Input: part model. Units: mm. Frame: model coordinates. A direction names the side the tool comes from. Coordinates: 2 decimals unless noted, no trailing zeros. Write each loop counter-clockwise with the first axis right and the second up, starting at its lowest first coordinate (ties: lowest second). Pieces come first, ordered by that corner, then holes. Notation, with made-up numbers: (40, 37.25) - (79, 37.25) arc R34 cw to (79, 76.25) - close; hole circle Ø11 at (44, -33). An arc over 180 degrees is marked (long way). One line per question, with ' | ' between items. Start each with the question number.
1) Reachability of faces 5 (the cylindrical face through (-1.55, 95.59, 14.84)), 6 (the cylindrical face through (13.836, 0.764, 7.924)) from +Z, -Z, +X, -X, +Y, -Y: full face, straight path, thin tool, end or side. Return the list, or none.
2) Section query A-A on y = 32.5. Return loops of the section in (x, z), and give its area (3 significant figures).
3) First-contact query: P1, Ø5, axis at y = 21.5, z = -6.5, coming from the -X side; P2, Ø2, axis at y = 54.5, z = 5, coming from the -X side; P3, Ø2, axis at x = -6, z = 3.5, coming from the +Y side. Flat tips, straight axial feed; report the tip coordinate or a pass-through.
4) Line query: line 1 (X direction, y = 49, z = 0); line 2 (Z direction, x = 3, y = 36.5); line 3 (Z direction, x = 14, y = 41). Output: solid intervals per line, ascending.
5) Draft query along Z for faces 1 (the cylindrical face through (-0.06, 0.76, -15.94)), 2 (the cylindrical face through (9.351, 49.811, 16.372)), 3 (the flat face through (-15.5, 98.425, -2.6)), 4 (the flat face through (0, 12.7, 0)). Return one class per face: released by +Z, released by -Z, zero draft, split by the parting line, or undercut.
```python
from build123d import *

# Parameters (mm, degrees)
BOSS_EXTRUDE1_DEPTH      = 98.425
SKETCH3_R                = 15.478125
CUT_EXTRUDE1_DEPTH       = 85.725
FILLET1_R                = 1.27
FILLET2_R                = 2.54
FILLET3_R                = 2.54
BOSS_EXTRUDE3_DEPTH      = 0.79375
BOSS_EXTRUDE3_DEPTH_BACK = 3.175
SKETCH7_R                = 1.5875
CUT_EXTRUDE2_START       = -0.635
SKETCH8_R                = 1.5875
CUT_EXTRUDE2_DEPTH       = 0.635
FILLET4_R                = 1.524
FILLET5_R                = 0.254


with BuildPart() as part:
    # Sketch2 → Boss-Extrude1 (new body)
    with BuildSketch(Plane(origin=(0, 0, 0), x_dir=(1, 0, 0), z_dir=(0, 1, 0))):
        Polygon((9.562214756, -16.704101823), (19.247283904, -0.070930017), (9.685069148, 16.633171806), (-9.562214756, 16.704101823), (-19.247283904, 0.070930017), (-9.685069148, -16.633171806), align=None)
    extrude(amount=BOSS_EXTRUDE1_DEPTH)

    # Sketch3 → Cut-Extrude1 (cut)
    with BuildSketch(Plane(origin=(0, 98.425, 0), x_dir=(1, 0, 0), z_dir=(0, 1, 0))):
        with Locations(Location((0, 0, 0), (0, 0, 270))):
            Circle(SKETCH3_R)
    extrude(amount=-CUT_EXTRUDE1_DEPTH, mode=Mode.SUBTRACT)

    # Fillet1
    fillet1_edges = [part.edges().sort_by_distance(p)[0] for p in [
        (0, 12.7, -15.478125),
    ]]
    fillet(fillet1_edges, radius=FILLET1_R)

    # Fillet2
    fillet2_edges = [part.edges().sort_by_distance(p)[0] for p in [
        (-14.466176526, 0, 8.281120895),
        (-14.40474933, 0, -8.38751592),
        (0.061427196, 0, -16.668636815),
        (14.466176526, 0, -8.281120895),
        (14.40474933, 0, 8.38751592),
        (-0.061427196, 0, 16.668636815),
    ]]
    fillet(fillet2_edges, radius=FILLET2_R)

    # Fillet3
    # the kernel refuses this fillet: 2.54 mm, written as the material it takes off along each edge
    with BuildSketch(Plane(origin=(-16.314364452, 2.54, -0.060121633), x_dir=(-0.8678621088062781, 0, 0.49680515305129436), z_dir=(0, -1, 0))) as fillet3_piece_1_section:
        Polygon((0, 0), (FILLET3_R, 0), (FILLET3_R, FILLET3_R * 0.57735026919), (FILLET3_R * 0.5, FILLET3_R * 0.866025403784), align=None)
    fillet3_piece_1 = extrude(amount=FILLET3_R, mode=Mode.PRIVATE)
    fillet3_piece_1 = fillet3_piece_1 - Plane(origin=(-16.314364452, 2.54, -0.060121633), x_dir=(0.9999932097338184, 0, 0.003685171129701924), z_dir=(0, -1, 0)) * Sphere(FILLET3_R, mode=Mode.PRIVATE)
    add(fillet3_piece_1, mode=Mode.SUBTRACT)
    with BuildSketch(Plane(origin=(-8.105115364, 2.54, -14.158714879), x_dir=(0.003685171129702339, 0, -0.9999932097338186), z_dir=(0, -1, 0))) as fillet3_piece_2_section:
        Polygon((0, 0), (FILLET3_R, 0), (FILLET3_R, -FILLET3_R * 0.57735026919), (FILLET3_R * 0.5, -FILLET3_R * 0.866025403784), align=None)
    fillet3_piece_2 = extrude(amount=FILLET3_R, mode=Mode.PRIVATE)
    fillet3_piece_2 = fillet3_piece_2 - Plane(origin=(-8.105115364, 2.54, -14.158714879), x_dir=(0.49680515305129425, 0, 0.867862108806278), z_dir=(0, -1, 0)) * Sphere(FILLET3_R, mode=Mode.PRIVATE)
    add(fillet3_piece_2, mode=Mode.SUBTRACT)
    with BuildSketch(Plane(origin=(-8.209249088, 2.54, 14.098593245), x_dir=(-0.003685171129702708, 0, 0.9999932097338186), z_dir=(0, -1, 0))) as fillet3_piece_3_section:
        Polygon((0, 0), (FILLET3_R, 0), (FILLET3_R, FILLET3_R * 0.57735026919), (FILLET3_R * 0.5, FILLET3_R * 0.866025403784), align=None)
    fillet3_piece_3 = extrude(amount=FILLET3_R, mode=Mode.PRIVATE)
    fillet3_piece_3 = fillet3_piece_3 - Plane(origin=(-8.209249088, 2.54, 14.098593245), x_dir=(0.5031880566825245, 0, -0.8641769376765759), z_dir=(0, -1, 0)) * Sphere(FILLET3_R, mode=Mode.PRIVATE)
    add(fillet3_piece_3, mode=Mode.SUBTRACT)
    with BuildSketch(Plane(origin=(8.209249088, 2.54, -14.098593245), x_dir=(0.8678621088062781, 0, -0.49680515305129436), z_dir=(0, -1, 0))) as fillet3_piece_4_section:
        Polygon((0, 0), (FILLET3_R, 0), (FILLET3_R, -FILLET3_R * 0.57735026919), (FILLET3_R * 0.5, -FILLET3_R * 0.866025403784), align=None)
    fillet3_piece_4 = extrude(amount=FILLET3_R, mode=Mode.PRIVATE)
    fillet3_piece_4 = fillet3_piece_4 - Plane(origin=(8.209249088, 2.54, -14.098593245), x_dir=(-0.5031880566825243, 0, 0.8641769376765759), z_dir=(0, -1, 0)) * Sphere(FILLET3_R, mode=Mode.PRIVATE)
    add(fillet3_piece_4, mode=Mode.SUBTRACT)
    with BuildSketch(Plane(origin=(8.105115364, 2.54, 14.158714879), x_dir=(0.8641769376765761, 0, 0.5031880566825242), z_dir=(0, -1, 0))) as fillet3_piece_5_section:
        Polygon((0, 0), (FILLET3_R, 0), (FILLET3_R, FILLET3_R * 0.57735026919), (FILLET3_R * 0.5, FILLET3_R * 0.866025403784), align=None)
    fillet3_piece_5 = extrude(amount=FILLET3_R, mode=Mode.PRIVATE)
    fillet3_piece_5 = fillet3_piece_5 - Plane(origin=(8.105115364, 2.54, 14.158714879), x_dir=(-0.4968051530512941, 0, -0.8678621088062782), z_dir=(0, -1, 0)) * Sphere(FILLET3_R, mode=Mode.PRIVATE)
    add(fillet3_piece_5, mode=Mode.SUBTRACT)
    with BuildSketch(Plane(origin=(16.314364452, 2.54, 0.060121633), x_dir=(0.8641769376765761, 0, 0.5031880566825242), z_dir=(0, -1, 0))) as fillet3_piece_6_section:
        Polygon((0, 0), (FILLET3_R, 0), (FILLET3_R, -FILLET3_R * 0.57735026919), (FILLET3_R * 0.5, -FILLET3_R * 0.866025403784), align=None)
    fillet3_piece_6 = extrude(amount=FILLET3_R, mode=Mode.PRIVATE)
    fillet3_piece_6 = fillet3_piece_6 - Plane(origin=(16.314364452, 2.54, 0.060121633), x_dir=(-0.9999932097338184, 0, -0.003685171129701988), z_dir=(0, -1, 0)) * Sphere(FILLET3_R, mode=Mode.PRIVATE)
    add(fillet3_piece_6, mode=Mode.SUBTRACT)
    with BuildSketch(Plane(origin=(-9.685069148, 2.54, 16.633171806), x_dir=(0.9999932097338186, 0, 0.0036851711297037465), z_dir=(0, 1, 0)), Plane(origin=(-19.247283904, 2.54, -0.070930017), x_dir=(0.49680515305129397, 0, 0.8678621088062782), z_dir=(0, 1, 0)), Plane(origin=(9.562214756, 2.54, 16.704101823), x_dir=(0.5031880566825245, 0, -0.8641769376765758), z_dir=(0, 1, 0))) as fillet3_piece_7:
        with BuildLine():
            CenterArc((FILLET3_R * 0.57735026919, FILLET3_R), FILLET3_R, 210, 60)
            Line((-FILLET3_R * 0.288675134595, FILLET3_R * 0.5), (0, 0))
            Line((0, 0), (FILLET3_R * 0.57735026919, 0))
        make_face()
    extrude(amount=99.551174209, mode=Mode.SUBTRACT)
    with BuildSketch(Plane(origin=(-9.562214756, 2.54, -16.704101823), x_dir=(0.9999932097338186, 0, 0.003685171129701324), z_dir=(0, 1, 0)), Plane(origin=(9.685069148, 2.54, -16.633171806), x_dir=(0.4968051530512946, 0, 0.8678621088062779), z_dir=(0, 1, 0)), Plane(origin=(19.247283904, 2.54, 0.070930017), x_dir=(-0.503188056682524, 0, 0.8641769376765761), z_dir=(0, 1, 0))) as fillet3_piece_8:
        with BuildLine():
            CenterArc((FILLET3_R * 0.57735026919, -FILLET3_R), FILLET3_R, 90, 60)
            Line((-FILLET3_R * 0.288675134595, -FILLET3_R * 0.5), (0, 0))
            Line((0, 0), (FILLET3_R * 0.57735026919, 0))
        make_face()
    extrude(amount=99.551174209, mode=Mode.SUBTRACT)

    # Sketch7 → Boss-Extrude3 (add, two sides: drawn at the far end of the back side and taken through both)
    with BuildSketch(Plane.XY.offset(15.478125).offset(-BOSS_EXTRUDE3_DEPTH_BACK)):
        with Locations(Location((0, 95.25, 0), (0, 0, 270))):
            Circle(SKETCH7_R)
    extrude(amount=BOSS_EXTRUDE3_DEPTH + BOSS_EXTRUDE3_DEPTH_BACK)

    # Sketch8 → Cut-Extrude2 (cut)
    with BuildSketch(Plane(origin=(0, 0, 12.303125), x_dir=(-1, 0, 0), z_dir=(0, 0, -1)).offset(CUT_EXTRUDE2_START)):
        with Locations((0, 95.25)):
            Circle(SKETCH8_R)
    extrude(amount=CUT_EXTRUDE2_DEPTH, mode=Mode.SUBTRACT)

    # Fillet4
    fillet4_edges = [part.edges().sort_by_distance(p)[0] for p in [
        (0, 96.8375, 12.938125),
    ]]
    fillet(fillet4_edges, radius=FILLET4_R)

    # Fillet5
    fillet5_edges = [part.edges().sort_by_distance(p)[0] for p in [
        (1.5875, 95.25, 15.396499513),
    ]]
    fillet(fillet5_edges, radius=FILLET5_R)


solid = part.part
```
Answer key:
1) face 5: none | face 6: +Z, +X, -Y
2) outline: (-18.52, 1.2) arc R2.54 ccw to (-18.51, -1.34) - (-10.3, -15.44) arc R2.54 ccw to (-8.1, -16.7) - (8.22, -16.64) arc R2.54 ccw to (10.41, -15.36) - (18.52, -1.2) arc R2.54 ccw to (18.51, 1.34) - (10.3, 15.44) arc R2.54 ccw to (8.1, 16.7) - (-8.22, 16.64) arc R2.54 ccw to (-10.41, 15.36) - close; hole circle Ø30.96 at (0, 0) | area: 208 mm²
3) P1: x = -16.96 | P2: x = -16.92 | P3: y = 12.7
4) line 1: -18.85 to -15.48, 15.48 to 18.85 | line 2: -16.66 to -15.18, 15.18 to 16.68 | line 3: -9.1 to -6.6, 6.6 to 9.08
5) face 1: released by -Z | face 2: released by +Z | face 3: zero draft | face 4: undercut
